Design review of the part shown in the three views and the two pictorial views. Dimensions are in mm from the part's minimum x, y and z. Coordinates: 2 decimals unless noted, no trailing zeros. Write each loop counter-clockwise with the first axis right and the second up, starting at its lowest first coordinate (ties: lowest second). Pieces come first, ordered by that corner, then holes. Notation, with made-up numbers: (56, 55) -> (104, 55) arc R16 ccw to (104, 83) -> close; hole circle Ø10 at (41, 66.25). An arc over 180 degrees is marked (long way). Answer in a Markdown table with one row per item. Add a question column.
Item 1: Take a section at C-C, the plane x = 70. Write out the cut boundary in (y, z).
Item 2: Draft analysis for pull direction X (two halves, no side actions). For the marked faces 1, 2 and 3, state which applies: released by +X, released by -X, zero draft, split by the parting line, or undercut.
Item 3: Take a section at B-B, the plane z = 27. Write out the cut boundary in (x, y), and give its area (3 significant figures).
Item 4: Take a section at A-A, the plane y = 60. Write out the cut boundary in (x, z).
Item 5: Clearance check with flat-ended pins moving along their axes: P1, Ø6, axis at y = 88.5, z = 52.5, coming from the -X side; P2, Ø1.5, axis at x = 39, z = 33.5, coming from the +Y side; P3, Ø4, axis at x = 51.5, z = 63, coming from the +Y side. State where each tip first meets the part, or that it passes through.
Item 6: To check wall thickness, follow line 1 (Y direction, x = 60, z = 50); line 2 (X direction, y = 58.5, z = 34); line 3 (Z direction, x = 49, y = 64.5). State the ranges of each line that lie inside material, in increasing order.
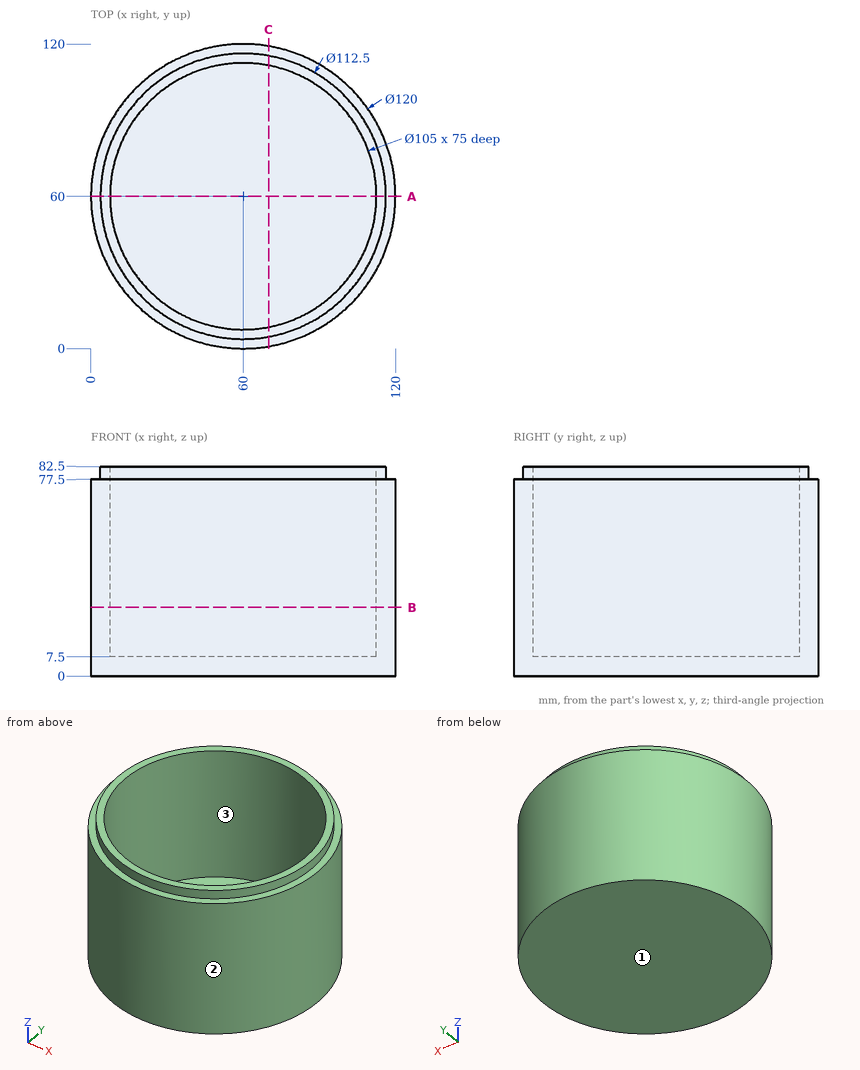
Answers:
| question | item | result |
|---|---|---|
| 1 | outline | (0.84, 0) -> (119.16, 0) -> (119.16, 77.5) -> (115.35, 77.5) -> (115.35, 82.5) -> (111.54, 82.5) -> (111.54, 7.5) -> (8.46, 7.5) -> (8.46, 82.5) -> (4.65, 82.5) -> (4.65, 77.5) -> (0.84, 77.5) -> close |
| 2 | face 1 | zero draft |
| 2 | face 2 | split by the parting line |
| 2 | face 3 | undercut |
| 3 | outline | circle Ø120 at (60, 60); hole circle Ø105 at (60, 60) |
| 3 | area | 2,650 mm^2 |
| 4 | outline | (0, 0) -> (120, 0) -> (120, 77.5) -> (116.25, 77.5) -> (116.25, 82.5) -> (112.5, 82.5) -> (112.5, 7.5) -> (7.5, 7.5) -> (7.5, 82.5) -> (3.75, 82.5) -> (3.75, 77.5) -> (0, 77.5) -> close |
| 5 | P1 | stops at x = 5.69 |
| 5 | P2 | stops at y = 116.48 |
| 5 | P3 | stops at y = 119.65 |
| 6 | line 1 | y = 0 to 7.5, 112.5 to 120 |
| 6 | line 2 | x = 0.02 to 7.52, 112.48 to 119.98 |
| 6 | line 3 | z = 0 to 7.5 |
